```python
from build123d import *

# Parameters (mm, degrees)
SALIENTE_EXTRUIR1_DEPTH = 19.3
CROQUIS2_W              = 15.3
CROQUIS2_H              = 26.3
CORTAR_EXTRUIR1_DEPTH   = 9.3
CORTAR_EXTRUIR2_DEPTH   = 12.3
CROQUIS6_R              = 0.75
SALIENTE_EXTRUIR2_DEPTH = 2
CROQUIS7_W              = 19.3
CROQUIS7_H              = 25
SALIENTE_EXTRUIR3_DEPTH = 3


with BuildPart() as part:
    # Croquis1 → Saliente-Extruir1 (new body)
    with BuildSketch(Plane.XY):
        with BuildLine():
            Line((5.8, 23.05), (2.4, 23.05))
            Line((2.4, 23.05), (-5.8, -0.85))
            Line((-5.8, -0.85), (-5.8, -10.609737321))
            ThreePointArc((-5.8, -10.609737321), (-5.505459406, -11.318487649), (-4.795345946, -11.609726491))
            Line((-4.795345946, -11.609726491), (-4.702327027, -11.609293571))
            ThreePointArc((-4.702327027, -11.609293571), (-4.347270297, -11.754912992), (-4.2, -12.109288156))
            Line((-4.2, -12.109288156), (-4.2, -21.05))
            ThreePointArc((-4.2, -21.05), (-3.614213562, -22.464213562), (-2.2, -23.05))
            Line((-2.2, -23.05), (-0.2, -23.05))
            ThreePointArc((-0.2, -23.05), (1.214213562, -22.464213562), (1.8, -21.05))
            Line((1.8, -21.05), (1.8, -13.106955688))
            ThreePointArc((1.8, -13.106955688), (2.239339828, -12.046295517), (3.3, -11.606955688))
            Line((3.3, -11.606955688), (3.8, -11.606955688))
            ThreePointArc((3.8, -11.606955688), (5.214213562, -11.021169251), (5.8, -9.606955688))
            Line((5.8, -9.606955688), (5.8, 23.05))
        make_face()
    extrude(amount=SALIENTE_EXTRUIR1_DEPTH)

    # Croquis2 → Cortar-Extruir1 (cut)
    with BuildSketch(Plane.ZY.offset(5.8)):
        with Locations((9.65, 9.9)):
            Rectangle(CROQUIS2_W, CROQUIS2_H)
    extrude(amount=-CORTAR_EXTRUIR1_DEPTH, mode=Mode.SUBTRACT)

    # Croquis4 → Cortar-Extruir2 (cut)
    with BuildSketch(Plane.ZY.offset(5.8)):
        Polygon((2.15, -5.239890457), (2.15, -6.239890457), (3.15, -6.239890457), (3.15, -7.239890457), (-0.05, -7.239890457), (-0.05, -23.239890457), (17.1, -23.239890457), (17.1, -7.239890457), (16.15, -7.239890457), (16.15, -6.239890457), (17.15, -6.239890457), (17.15, -5.239890457), align=None)
    extrude(amount=-CORTAR_EXTRUIR2_DEPTH, mode=Mode.SUBTRACT)

    # Croquis6 → Saliente-Extruir2 (add)
    with BuildSketch(Plane.XY.offset(19.3)):
        with Locations((-0.655214383, -15.046201441)):
            Circle(CROQUIS6_R)
    extrude(amount=SALIENTE_EXTRUIR2_DEPTH)

    # Croquis7 → Saliente-Extruir3 (add)
    with BuildSketch(Plane(origin=(5.8, 0, 0), x_dir=(0, 0, -1), z_dir=(1, 0, 0))):
        with Locations((-9.65, 10.55)):
            Rectangle(CROQUIS7_W, CROQUIS7_H)
    extrude(amount=SALIENTE_EXTRUIR3_DEPTH)


solid = part.part
```
Geometry check sheet. Reference: the model listing, model coordinates, mm. A direction names the side the tool comes from. Give positions to 0.01 mm unless a question says otherwise; leave off trailing zeros. Order: outer loops, then holes, each group sorted by start corner. A loop starts at its lowest first (then second) coordinate and runs counter-clockwise, first axis right, second up.
1. Section check D-D, the plane y = -19. Enter the section's corners in (x, z).
2. Access from +Z, -Z, +X, -X, +Y, -Y to the whole of each face (thin tool, end or side, straight path). Record for faces 1 (the face through (-0.1, -7.24, 16.6)), 2 (the face through (0, -7, 16.15)), 3 (the face through (0, 7, 17.3)), 4 (the face through (-4.2, -17, 18)), 5 (the face through (1.8, -17, 18)).
3. Gauge pin test, flat ends, axial feed: pin 1 Ø10 at (y, z) = (17, 18.5) entering from -X; pin 2 Ø10 at (y, z) = (4.5, 2.5) entering from -X; pin 3 Ø2.5 at (x, z) = (7.5, 8.5) entering from -Y. Record the tip position at first contact, or that the pin passes through.
4. Section check C-C, the plane x = 4.25. Enter the section's corners in (y, z), and give its area (3 significant figures).
5. Thickness scan on L1, parallel to Y at x = 7.25, z = 8.5; L2, parallel to X at y = 3, z = 11.75; L3, parallel to Y at x = 1, z = 3. Record the ranges inside material, lowest first.
6. Section check B-B, the plane y = 15. Enter the section's corners in (x, z).
7. Section check A-A, the plane z = 9.5. Enter the section's corners in (x, y), and give its area (3 significant figures).
Values follow:
1. outline: (-4.2, 17.1) - (1.8, 17.1) - (1.8, 19.3) - (-4.2, 19.3) - close
2. face 1: -Z, +X, -X, -Y
2. face 2: +X, -X, -Y
2. face 3: -X, +Y
2. face 4: +Z, -Z, -X, -Y
2. face 5: +Z, -Z, +X, -Y
3. pin 1: stops at x = -1.39
3. pin 2: stops at x = -5.67
3. pin 3: stops at y = -1.95
4. outline: (-11.56, 17.1) - (-7.24, 17.1) - (-7.24, 16.15) - (-6.24, 16.15) - (-6.24, 17.15) - (-5.24, 17.15) - (-5.24, 2.15) - (-6.24, 2.15) - (-6.24, 3.15) - (-7.24, 3.15) - (-7.24, 0) - (23.05, 0) - (23.05, 19.3) - (-11.56, 19.3) - close
4. area: 566 mm2
5. L1: y = -1.95 to 23.05
5. L2: x = 3.5 to 8.8
5. L3: y = -7.24 to -6.24, -5.24 to -3.25
6. outline: (-0.36, 0) - (8.8, 0) - (8.8, 19.3) - (-0.36, 19.3) - (-0.36, 17.3) - (3.5, 17.3) - (3.5, 2) - (-0.36, 2) - close
7. outline: (-5.8, -5.24) - (5.8, -5.24) - (5.8, -1.95) - (8.8, -1.95) - (8.8, 23.05) - (3.5, 23.05) - (3.5, -3.25) - (-5.8, -3.25) - close
7. area: 159 mm2
